Geometry: final body of the model. Coordinates: model frame, mm. A direction names the side the tool comes from. Give positions to 0.01 mm unless a question says otherwise; leave off trailing zeros. Write each loop counter-clockwise with the first axis right and the second up, starting at its lowest first coordinate (ties: lowest second). Pieces come first, ordered by that corner, then holes.
Q1. Draft query along Z for faces 3 (the face through (11, -0.1, -2.5)), 4 (the face through (21.09, 0, 0)), 5 (the face through (0.545, 0, 0)). Return one class per face: pulls with the +Z half, pulls with the -Z half, needs draft (parallel to the pull), parting line crosses it, or undercut.
Q2. Reachability of faces 1 (the face through (0, 2, -2)), 2 (the face through (1.09, 2, 2)) from +Z, -Z, +X, -X, +Y, -Y: full face, straight path, thin tool, end or side. Return the list, or none.
Q3. Cut plane A-A on x = 8.75. Return the cut outline in (y, z).
Q4. Line query: L1, parallel to X at y = -2, z = 2.5; L2, parallel to Y at x = 16, z = 0; L3, parallel to Y at x = 14, z = 1.5. Output: solid intervals per line, ascending.
Q5. Pin query (flat end, axial travel): pin 1 (1.5 mm diameter, centred on x = 17.5, y = -2.5, fed in from -Z); pin 2 (2.5 mm diameter, centred on y = -1, z = 0.5, fed in from -X); pin 3 (2 mm diameter, centred on x = 7, y = -1, fed in from +Z); pin 4 (3 mm diameter, centred on x = 15.5, y = 3, fed in from +Z). Return the tip coordinate at first contact, or that it passes through.
```python
from build123d import *

# Parameters (mm, degrees)
CLINCHCUT_DEPTH    = 0.4905
CLINCHCUTPAT_COUNT = 24
CLINCHCUTPAT_ANGLE = 345


with BuildPart() as part:
    # BodySke → BaseBody (revolve)
    with BuildSketch(Plane.XY, mode=Mode.PRIVATE) as basebody_sk:
        Polygon((0, 2.2225), (0, 3.95), (0.1778, 3.95), (0.4905, 3.6373), (0.5995, 3.6373), (0.5995, 4.445), (1.09, 4.445), (1.09, 2.5), (20.645, 2.5), (21.09, 2.055), (21.09, 0), (0.545, 0), (0.545, 1.6775), align=None)
    revolve(basebody_sk.sketch.rotate(Axis((0, 0, 0), (1, 0, 0)), 90), axis=Axis((0, 0, 0), (1, 0, 0)))

    # CliRinCutSke → ClinchCut (cut)
    with BuildSketch(Plane(origin=(1.09, 0, 0), x_dir=(0, 0, -1), z_dir=(1, 0, 0))):
        with BuildLine():
            Line((0.580188924, 4.406972409), (0, 4.0005))
            Line((0, 4.0005), (-0.580188924, 4.406972409))
            ThreePointArc((-0.580188924, 4.406972409), (0, 4.445), (0.580188924, 4.406972409))
        make_face()
    clinchcut = extrude(amount=-CLINCHCUT_DEPTH, mode=Mode.SUBTRACT)

    # ClinchCutPat: ClinchCut ×24 about axis
    clinchcutpat_axis = Axis((0, 0, 0), (1, 0, 0))
    for i in range(1, CLINCHCUTPAT_COUNT):
        add(clinchcut.rotate(clinchcutpat_axis, i * CLINCHCUTPAT_ANGLE / (CLINCHCUTPAT_COUNT - 1)), mode=Mode.SUBTRACT)


solid = part.part
```
Data:
1. face 3: parting line crosses it
1. face 4: needs draft
1. face 5: undercut
2. face 1: +Z, -Z, -X, +Y, -Y
2. face 2: +X
3. outline: circle Ø5 at (0, 0)
4. L1: x = 0 to 1.09
4. L2: y = -2.5 to 2.5
4. L3: y = -2 to 2
5. pin 1: stops at z = -1.79
5. pin 2: stops at x = 0
5. pin 3: stops at z = 2.5
5. pin 4: stops at z = 2
